Geometry: final body of the model. Coordinates: model frame, mm. A direction names the side the tool comes from. Give positions to 0.01 mm unless a question says otherwise; leave off trailing zeros. Order: outer loops, then holes, each group sorted by start corner. A loop starts at its lowest first (then second) coordinate and runs counter-clockwise, first axis right, second up. Notation, with made-up numbers: (19.25, -37) - (26.25, -37) arc R31 ccw to (26.25, -6) - close; hole circle Ø10 at (58, 41.5). An arc over 180 degrees is marked (long way). One line per item, written item: value.
```python
from build123d import *

# Parameters (mm, degrees)
F0_R     = 1.5
F1_DEPTH = 1
F2_R     = 2


with BuildPart() as f1:
    # F0 (on Right) → F1 (new body)
    with BuildSketch(Plane.YZ):
        with BuildLine():
            Line((-12.25, 15), (-15.25, 15))
            Line((-15.25, 15), (-11.409494, 8.348048))
            ThreePointArc((-11.409494, 8.348048), (-15, 0), (-11.409494, -8.348048))
            Line((-11.409494, -8.348048), (-15.25, -15))
            Line((-15.25, -15), (-12.25, -15))
            Line((-12.25, -15), (-12.25, -16.5))
            Line((-12.25, -16.5), (-7.25, -16.5))
            Line((-7.25, -16.5), (-7.25, -15))
            Line((-7.25, -15), (-4.25, -15))
            Line((-4.25, -15), (-2.185775, -11.424658))
            ThreePointArc((-2.185775, -11.424658), (6.543653, -5.601343), (6.910541, 4.88576))
            Line((6.910541, 4.88576), (12.75, 15))
            Line((12.75, 15), (9.75, 15))
            Line((9.75, 15), (9.75, 16.5))
            Line((9.75, 16.5), (4.75, 16.5))
            Line((4.75, 16.5), (4.75, 15))
            Line((4.75, 15), (1.75, 15))
            Line((1.75, 15), (0.482051, 12.803848))
            ThreePointArc((0.482051, 12.803848), (-1.25, 11.803848), (-2.982051, 12.803848))
            Line((-2.982051, 12.803848), (-4.25, 15))
            Line((-4.25, 15), (-7.25, 15))
            Line((-7.25, 15), (-7.25, 16.5))
            Line((-7.25, 16.5), (-12.25, 16.5))
            Line((-12.25, 16.5), (-12.25, 15))
        make_face()
        with Locations((-3.5, 0)):
            Circle(F0_R, mode=Mode.SUBTRACT)
    extrude(amount=F1_DEPTH)

    # F2
    f2_edges = [f1.edges().sort_by_distance(p)[0] for p in [
        (0.5, -11.409494, 8.348048),
        (0.5, -11.409494, -8.348048),
        (0.5, -2.185775, -11.424658),
        (0.5, 6.910541, 4.88576),
    ]]
    fillet(f2_edges, radius=F2_R)


solid = f1.part
```
1) Section D-D, the plane z = -5.5. Return loops of the section in (x, y), then the cut area to 3 significant figures.
Answers below:
outline: (0, -13.6) - (1, -13.6) - (1, 6.6) - (0, 6.6) - close
area: 20.2 mm^2
2) First-contact query: pin 1 (8 mm diameter, centred on y = 2, z = 1.5, fed in from -X); pin 2 (0.5 mm diameter, centred on x = 0.5, z = 16, fed in from -Y). Flat tips, straight axial feed; report the tip coordinate or a pass-through.
Answers below:
pin 1: x = 0
pin 2: y = -12.25
3) Material intervals for line 1 along Z through (x, y) = (0.1, -7); line 2 along Z through (x, y) = (0.6, -3.5); line 3 along Y through (x, z) = (0.45, -3), sorted ascending.
Answers below:
line 1: -15 to 15
line 2: -13.7 to -1.5, 1.5 to 13.7
line 3: -14.6 to 7.6
4) Set-up query: faces 1 (the face through (0.5, -12.25, 15.8)), 2 (the face through (0.5, 9.75, 15.7)), 3 (the face through (0.49, -13.72, 12.35)). Return all of +Z, -Z, +X, -X, +Y, -Y with unobstructed straight access to the full face (end or side cutting, diameter ignored); none if empty.
Answers below:
face 1: +Z, +X, -X, -Y
face 2: +Z, +X, -X, +Y
face 3: +X, -X, -Y
5) Section A-A, the plane z = 0. Return loops of the section in (x, y), then the cut area to 3 significant figures.
Answers below:
outline: (0, -15) - (1, -15) - (1, -5) - (0, -5) - close; (0, -2) - (1, -2) - (1, 8) - (0, 8) - close
area: 20.0 mm^2
6) Mould query, pull axis Y, two halves, no side actions, for faces 4 (the face through (0.5, -7.25, 15.7)), 5 (the face through (0.49, -13.68, -12.28)), 6 (the face through (0.5, 7.3, 16.5)). Classes: released by +Y, released by -Y, zero draft, split by the parting line, or undercut.
Answers below:
face 4: undercut
face 5: released by -Y
face 6: zero draft
7) Section B-B, the plane y = -3.5. Return loops of the section in (x, z), then the cut area to 3 significant figures.
Answers below:
outline: (0, -13.7) - (1, -13.7) - (1, -1.5) - (0, -1.5) - close; (0, 1.5) - (1, 1.5) - (1, 13.7) - (0, 13.7) - close
area: 24.4 mm^2
